from build123d import *

# Parameters (mm, degrees)
F0_R           = 9.1313
F1_DEPTH       = 3.175
F3_DEPTH       = 1.524
F4_R           = 9.1313
F5_DEPTH       = 1.524
F6_R           = 9.1313
F7_DEPTH       = 1.651
F8_R           = 7.6073
F9_DEPTH       = 4.826
F10_R          = 0.635
F11_DEPTH      = 25.4
F11_DEPTH_BACK = 25.4
F12_R          = 1.27
F13_R          = 1.27


with BuildPart() as f1:
    # F0 (on Front) → F1 (new body)
    with BuildSketch(Plane.XZ):
        Circle(F0_R)
    extrude(amount=F1_DEPTH)

    # F2 (on face) → F3 (join)
    with BuildSketch(Plane.XZ.offset(3.175)):
        with BuildLine():
            Line((8.12546, 6.35), (-8.12546, 6.35))
            ThreePointArc((-8.12546, 6.35), (-10.3124, 0), (-8.12546, -6.35))
            Line((-8.12546, -6.35), (8.12546, -6.35))
            ThreePointArc((8.12546, -6.35), (10.3124, 0), (8.12546, 6.35))
        make_face()
    extrude(amount=F3_DEPTH)

    # F4 (on face) → F5 (join)
    with BuildSketch(Plane.XZ.offset(4.699)):
        Circle(F4_R)
    extrude(amount=-F5_DEPTH)

    # F6 (on face) → F7 (join)
    with BuildSketch(Plane.XZ.offset(4.699)):
        Circle(F6_R)
    extrude(amount=F7_DEPTH)

    # F8 (on face) → F9 (cut)
    with BuildSketch(Plane(origin=(0, 0, 0), x_dir=(-1, 0, 0), z_dir=(0, 1, 0))):
        Circle(F8_R)
    extrude(amount=-F9_DEPTH, mode=Mode.SUBTRACT)

    # F10 (on face) → F11 (cut, two sides)
    with BuildSketch(Plane.XZ.offset(6.35)) as f11_sk:
        Circle(F10_R)
    extrude(amount=-F11_DEPTH, mode=Mode.SUBTRACT)
    extrude(f11_sk.sketch, amount=-F11_DEPTH_BACK, mode=Mode.SUBTRACT)

    # F12
    f12_edges = [f1.edges().sort_by_distance(p)[0] for p in [
        (-9.1313, -6.35, 0),
    ]]
    fillet(f12_edges, radius=F12_R)

    # F13
    f13_edges = [f1.edges().sort_by_distance(p)[0] for p in [
        (-9.1313, 0, 0),
    ]]
    fillet(f13_edges, radius=F13_R)


solid = f1.part
Build history of the part. All positions in model axes, mm. A direction names the side the tool comes from. Coordinates: 2 decimals unless noted, no trailing zeros. Write each loop counter-clockwise with the first axis right and the second up, starting at its lowest first coordinate (ties: lowest second). Pieces come first, ordered by that corner, then holes.
(1) Drill centre lines: line 1 (Z direction, x = 0, y = -3.45); line 2 (Y direction, x = -1, z = 6.25); line 3 (Y direction, x = 9.5, z = -3.25) (3 decimals). Where is each one in solid material? Low to high.
(2) 3-axis set-ups, long thin cutter, end or side, ignore diameter. For faces 5 (the flat face through (-7, -4, 6.35)), 6 (the flat face through (-9.3, -4.699, 0)), 7 (the cylindrical face through (-7.256, -2.379, 2.285)), 8 (the flat face through (7, -4, 6.35)): which of +Z, -Z, +X, -X, +Y, -Y reach the whole face in a straight line?
(3) Cut at B-B on y = -1. List the corners of the cut face in (x, z).
(4) Cut at A-A on x = 0. List the corners of the cut face in (y, z) (3 decimals), and give its area (3 significant figures).
(5) Mould opens along Z. For faces 1 (the flat face through (0, -4.826, -2)), 2 (the flat face through (9.3, -3.175, 0.5)), 3 (the cylindrical face through (-0.08, -5.6, 0.63)), 4 (the flat face through (-7, -4, -6.35)) say: pulls with the +Z half, pulls with the -Z half, needs draft (parallel to the pull), parting line crosses it, or undercut.
(6) Pin check, flat tips, straight feed: pin 1 Ø4.5 at (x, z) = (-0.5, -0.5) entering from +Y; pin 2 Ø0.8 at (x, y) = (-7.5, -4) entering from +Z; pin 3 Ø0.5 at (x, y) = (7, -4) entering from -Z. Stop position of each tip, or through.
Working result:
1. line 1: z = -9.13 to -7.61, 7.61 to 9.13
1. line 2: y = -6.35 to -4.83
1. line 3: y = -4.699 to -3.175
2. face 5: +Z, -X, +Y, -Y
2. face 6: -X, -Y
2. face 7: +Y
2. face 8: +Z, +X, +Y, -Y
3. outline: circle Ø18.2 at (0, 0); hole circle Ø15.21 at (0, 0)
4. outline: (-6.35, -7.861) arc R1.27 ccw to (-5.08, -9.131) - (-1.27, -9.131) arc R1.27 ccw to (0, -7.861) - (0, -7.607) - (-4.826, -7.607) - (-4.826, -0.635) - (-6.35, -0.635) - close; (-6.35, 0.635) - (-4.826, 0.635) - (-4.826, 7.607) - (0, 7.607) - (0, 7.861) arc R1.27 ccw to (-1.27, 9.131) - (-5.08, 9.131) arc R1.27 ccw to (-6.35, 7.861) - close
4. area: 39.2 mm2
5. face 1: undercut
5. face 2: needs draft
5. face 3: undercut
5. face 4: pulls with the -Z half
6. pin 1: stops at y = -4.83
6. pin 2: stops at z = 6.35
6. pin 3: stops at z = -6.35
